```python
from build123d import *

# Parameters (mm, degrees)
BOSS_EXTRU_1_DEPTH    = 20
CONG_1_R              = 5
TROU_TARAUD_M51_D     = 4.2
TROU_TARAUD_M51_DEPTH = 25
TROU_TARAUD_M51_TIP   = 1.2618073


with BuildPart() as part:
    # Esquisse1 → Boss.-Extru.1 (new, symmetric)
    with BuildSketch(Plane.XY):
        Polygon((-20, 15), (-20, -35), (-10, -35), (-10, -30), (10, -30), (10, -10), (30, -10), (30, 0), (-10, 0), (-10, 15), align=None)
    extrude(amount=BOSS_EXTRU_1_DEPTH, both=True)

    # Congé1
    cong_1_edges = [part.edges().sort_by_distance(p)[0] for p in [
        (-10, -30, 0),
        (10, -10, 0),
        (10, -30, 0),
    ]]
    fillet(cong_1_edges, radius=CONG_1_R - 0.0001)  # a hair under: the kernel refuses the full size

    # Trou taraudé M51
    with Locations(Plane(origin=(0, 0, 0), x_dir=(1, 0, 0), z_dir=(0, 1, 0))):
        with Locations((0, 0)):
            Hole(TROU_TARAUD_M51_D / 2, depth=TROU_TARAUD_M51_DEPTH)
            with Locations((0, 0, -(TROU_TARAUD_M51_DEPTH + TROU_TARAUD_M51_TIP / 2))):  # 118° drill point
                Cone(0, TROU_TARAUD_M51_D / 2, TROU_TARAUD_M51_TIP, mode=Mode.SUBTRACT)


solid = part.part
```
Model file for the job. Use its own axes, mm. A direction names the side the tool comes from. Give positions to 0.01 mm unless a question says otherwise; leave off trailing zeros. Loops run counter-clockwise (first coordinate to the right, second up) from the corner with the lowest first, then second, coordinate; pieces in that order, holes last. Notation, with made-up numbers: (10.5, 21.25) - (63.5, 21.25) arc R22 cw to (63.5, 32.25) - close; hole circle Ø4 at (25.5, 29). An arc over 180 degrees is marked (long way). One line per item, written item: value. Start each with the question number.
1. Probe L1, parallel to Z at x = 0, y = -5.75; L2, parallel to Y at x = 22.5, z = 7; L3, parallel to X at y = -14, z = -0.5. List the from-to ranges inside material, lowest first. Write a range as from..to.
2. Pull direction Z, two halves, no side cores. Call faces 4 (the flat face through (10, 0, 0)), 5 (the conical face through (0.35, -26.04, -0.11)), 6 (the flat face through (-1, -10, -20)), 7 (the cylindrical face through (-2.003, -12.675, -0.631)): pulls with the +Z half, pulls with the -Z half, needs draft (parallel to the pull), parting line crosses it, or undercut.
3. Slice it at B-B (x = 26). List the corners of the cut face in (y, z).
4. Which spindle directions (+Z, -Z, +X, -X, +Y, -Y) get a long thin tool onto all of the face, cutting with end or side? Do faces 1 (the flat face through (-15, 15, 0)), 2 (the flat face through (10, -20, 0)), 3 (the flat face through (-10, 7, 0)). Say none if no direction does.
5. Pin check, flat tips, straight feed: pin 1 (12 mm diameter, centred on x = 22.5, z = 1, fed in from -Y); pin 2 (3.5 mm diameter, centred on x = 0, z = 0, fed in from -Y); pin 3 (11 mm diameter, centred on x = -1.5, z = 1, fed in from -Y). Stop position of each tip, or through.
6. Slice it at C-C (y = 3). List the corners of the cut face in (x, z).
Solution:
1. L1: z = -20..-2.1, 2.1..20
1. L2: y = -10..0
1. L3: x = -20..-2.04, 2.04..10.1
2. face 4: needs draft
2. face 5: undercut
2. face 6: pulls with the -Z half
2. face 7: undercut
3. outline: (-10, -20) - (0, -20) - (0, 20) - (-10, 20) - close
4. face 1: +Z, -Z, +X, -X, +Y
4. face 2: +Z, -Z, +X, -Y
4. face 3: +Z, -Z, +X, +Y
5. pin 1: stops at y = -10
5. pin 2: stops at y = -30
5. pin 3: stops at y = -30.42
6. outline: (-20, -20) - (-10, -20) - (-10, 20) - (-20, 20) - close
